```python
from build123d import *

# Parameters (mm, degrees)
BOSS_EXTRUDE2_DEPTH = 0.9
CIRPATTERN1_COUNT   = 6
CUT_REVOLVE2_ANGLE  = 18.3


with BuildPart() as part:
    # Sketch3 → Revolve2 (revolve)
    with BuildSketch(Plane(origin=(0, 0, 0), x_dir=(0, 0, -1), z_dir=(1, 0, 0))):
        with BuildLine():
            Line((5.4, 0), (5.4, 17.5))
            Line((5.4, 17.5), (6.250057305, 17.5))
            ThreePointArc((6.250057305, 17.5), (6.953368941, 17.789118334), (7.25, 18.489294515))
            Line((7.25, 18.489294515), (7.4, 32.5))
            Line((7.4, 32.5), (9.4, 34))
            Line((9.4, 34), (9.4, 77.7))
            Line((9.4, 77.7), (14.65, 77.7))
            Line((14.65, 77.7), (14.65, 79.2))
            Line((14.65, 79.2), (10.75, 79.2))
            Line((10.75, 79.2), (10.75, 87))
            Line((10.75, 87), (9.5, 87))
            Line((9.5, 87), (9.5, 79))
            Line((9.5, 79), (8.1, 77))
            Line((8.1, 77), (8.1, 34))
            Line((8.1, 34), (6, 32.425))
            Line((6, 32.425), (5.856270621, 19))
            Line((5.856270621, 19), (2.539122418, 14.6))
            Line((2.539122418, 14.6), (2.1, 11.5))
            Line((2.1, 11.5), (2.85, 11.5))
            Line((2.85, 11.5), (3.062478589, 13))
            Line((3.062478589, 13), (3.75, 13))
            Line((3.75, 13), (3.75, 2))
            Line((3.75, 2), (4.4, 0))
            Line((4.4, 0), (5.4, 0))
        make_face()
    revolve(axis=Axis((0, 0, 0), (0, 1, 0)))

    # Sketch4 → Boss-Extrude2 (add)
    with BuildSketch(Plane(origin=(0, 0, 0), x_dir=(0, 0, -1), z_dir=(1, 0, 0))):
        with BuildLine():
            Line((8.5, 34.3), (8.308857775, 16.446417237))
            ThreePointArc((8.308857775, 16.446417237), (8.025083083, 15.776587579), (7.352253864, 15.5))
            Line((7.352253864, 15.5), (3.217630005, 15.5))
            Line((3.217630005, 15.5), (5.856270621, 19))
            Line((5.856270621, 19), (6, 32.425))
            Line((6, 32.425), (8.5, 34.3))
        make_face()
    boss_extrude2 = extrude(amount=BOSS_EXTRUDE2_DEPTH)

    # CirPattern1: Boss-Extrude2 ×6 about axis
    cirpattern1_axis = Axis((0, 0, 0), (0, 1, 0))
    for i in range(1, CIRPATTERN1_COUNT):
        add(boss_extrude2.rotate(cirpattern1_axis, i * 360 / CIRPATTERN1_COUNT))

    # Sketch6 → Cut-Revolve2 (revolve, symmetric, cut)
    with BuildSketch(Plane(origin=(0, 0, 0), x_dir=(0, 0, -1), z_dir=(1, 0, 0))) as cut_revolve2_sk:
        Polygon((8.1, 77), (8.1, 72.4), (9.5, 73.6), (9.5, 79), align=None)
    revolve(axis=Axis((0, 0, 0), (0, 1, 0)), revolution_arc=CUT_REVOLVE2_ANGLE / 2, mode=Mode.SUBTRACT)
    revolve(cut_revolve2_sk.sketch, axis=Axis((0, 0, 0), (0, -1, 0)), revolution_arc=CUT_REVOLVE2_ANGLE / 2, mode=Mode.SUBTRACT)


solid = part.part
```
Input: part model. Units: mm. Frame: model coordinates. A direction names the side the tool comes from. Coordinates: 2 decimals unless noted, no trailing zeros. Write each loop counter-clockwise with the first axis right and the second up, starting at its lowest first coordinate (ties: lowest second). Pieces come first, ordered by that corner, then holes. Notation, with made-up numbers: (62.25, 66) - (72.25, 66) arc R23 cw to (72.25, 105) - close; hole circle Ø1 at (-2, 77.5). An arc over 180 degrees is marked (long way). Put each result on its own line as item: value. Start each with the question number.
1) Ray query, L1, parallel to Z at x = 0, y = 85.5; L2, parallel to Z at x = 0, y = 5. Return the intervals inside material, ascending.
2) Mould query, pull axis X, two halves, no side actions, for faces 5 (the face through (-0.347, 77.319, 8.316)), 6 (the face through (-6, 17.5, 0)), 7 (the face through (-3, 17.5, 5)), 8 (the face through (7.31, 25.59, 0.49)). Classes: pulls with the +X half, pulls with the -X half, needs draft (parallel to the pull), parting line crosses it, or undercut.
3) Cut plane B-B (x = 12.25). Return the cut outline in (y, z), plus the area to 3 significant figures.
4) Cut plane C-C (y = 53.5). Return the cut outline in (x, z).
5) Cut plane A-A (y = 8). Return the cut outline in (x, z).
6) Reachability of faces 1 (the face through (-8, 79.2, 8)), 2 (the face through (6, 15.5, -3)), 3 (the face through (0, 23, -8)), 4 (the face through (0, 23, 8)) from +Z, -Z, +X, -X, +Y, -Y: full face, straight path, thin tool, end or side. Return the list, or none.
7) Contact query for flat-ended pins moving along their axis: pin 1 (3 mm diameter, centred on x = 2.5, z = 4.5, fed in from -Y); pin 2 (3.5 mm diameter, centred on y = 28, z = 7.5, fed in from +X); pin 3 (2 mm diameter, centred on x = -4, y = 70, fed in from -Z); pin 4 (1.4 mm diameter, centred on x = -5, z = -4, fed in from -Y). Output: stop coordinate, or through.
Resolved:
1. L1: z = -10.75 to -9.5, 9.5 to 10.75
1. L2: z = -5.4 to -3.75, 3.75 to 5.4
2. face 5: undercut
2. face 6: needs draft
2. face 7: undercut
2. face 8: pulls with the +X half
3. outline: (77.7, -8.03) - (79.2, -8.03) - (79.2, 8.03) - (77.7, 8.03) - close
3. area: 24.1 mm2
4. outline: circle Ø18.8 at (0, 0); hole circle Ø16.2 at (0, 0)
5. outline: circle Ø10.8 at (0, 0); hole circle Ø7.5 at (0, 0)
6. face 1: +Y
6. face 2: -Z, +X, -Y
6. face 3: -Z, -X, -Y
6. face 4: +Z, +X, -Y
7. pin 1: stops at y = 0
7. pin 2: stops at x = 4.58
7. pin 3: stops at z = -8.91
7. pin 4: stops at y = 15.5
